Could you check a few things on this drawing? It's one solid part, dimensions in mm from its lowest x, y, z. A direction names the side the tool comes from. Round coordinates to 2 decimals unless told otherwise and drop trailing zeros. Loops run counter-clockwise (first coordinate to the right, second up) from the corner with the lowest first, then second, coordinate; pieces in that order, holes last. Notation, with made-up numbers: M 68.5,85.25 L 124.5,85.25 A16 cw 124.5,103.25 Z; hole C 7.25,70.5 d2. An arc over 180 degrees is marked long. Use a Markdown table: item, result. Add a question column.
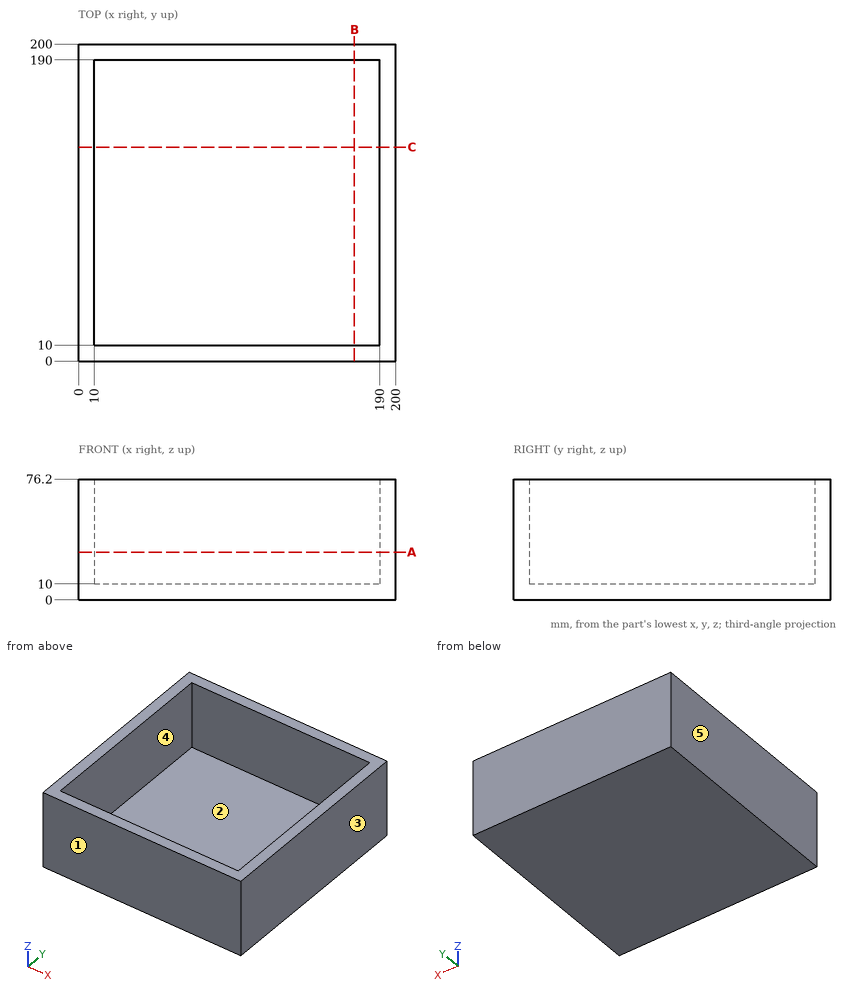
(1) On a 3-axis mill with a long thin cutter (end or side, diameter ignored), from which of +Z, -Z, +X, -X, +Y, -Y can I reach the whole of each face in a straight line? I mean the marked faces 1 and 2. Say none if no direction works.
(2) I'm going to push a flat-ended pin straight in: pin 1 (10 mm diameter, centred on x = 119, y = 80, fed in from +Z). Where does the tip first touch, or does it pass through?
(3) If I drill on probe 1 along Y at (x, z) = (12.5, 34); probe 2 along Z at (x, y) = (164, 149.5), over which ranges is the centre line in solid material (lowest first)? Write a range as [from, to].
(4) Thinking about a two-plate mould opening in X: for the marked faces 3, 4 and 5, which applies, released by +X, released by -X, zero draft, split by the parting line, or undercut?
(5) Suppose I cut it at A-A on z = 30. List the corners of the cut face in (x, y) for me.
(6) Suppose I cut it at B-B on x = 174. List the corners of the cut face in (y, z) for me.
Results below:
| question | item | result |
|---|---|---|
| 1 | face 1 | +Z, -Z, +X, -X, -Y |
| 1 | face 2 | +Z |
| 2 | pin 1 | stops at z = 10 |
| 3 | probe 1 | y = [0, 10], [190, 200] |
| 3 | probe 2 | z = [0, 10] |
| 4 | face 3 | released by +X |
| 4 | face 4 | undercut |
| 4 | face 5 | released by -X |
| 5 | outline | M 0,0 L 200,0 L 200,200 L 0,200 Z; hole M 10,10 L 190,10 L 190,190 L 10,190 Z |
| 6 | outline | M 0,0 L 200,0 L 200,76.2 L 190,76.2 L 190,10 L 10,10 L 10,76.2 L 0,76.2 Z |
